For this review, take the finished solid that the model builds, in its own axes (mm). A direction names the side the tool comes from. Coordinates: 2 decimals unless noted, no trailing zeros. Write each loop counter-clockwise with the first axis right and the second up, starting at its lowest first coordinate (ties: lowest second). Pieces come first, ordered by that corner, then holes. Notation, with made-up numbers: (36, 50.25) -> (44, 50.25) arc R20 ccw to (44, 69.25) -> close; hole circle Ø8 at (58, 87.5). An arc over 180 degrees is marked (long way). Put each result on its own line as item: value. Start each with the question number.
Item 1: Consider section B-B on y = -3.5. Give the boundary of the cut face in (x, z), and give its area (3 significant figures).
Item 2: Consider section C-C on z = -97.5. Give the boundary of the cut face in (x, y), and give its area (3 significant figures).
Item 3: To check wall thickness, follow L1, parallel to Y at x = 125, z = -45; L2, parallel to Z at x = 26, y = -8.5; L3, parallel to Y at x = 14, z = -9. State the ranges of each line that lie inside material, in increasing order.
Item 4: Consider section A-A on x = 125.5. Give the boundary of the cut face in (y, z), and give its area (3 significant figures).
Item 5: Consider section D-D on x = 147. Give the boundary of the cut face in (y, z), and give its area (3 significant figures).
Item 6: Insertion check: P1, Ø6, axis at x = 101, y = -26, coming from the -Z side; P2, Ø6, axis at x = 33.5, z = -93.5, coming from the -Y side; P3, Ø5, axis at x = 147.5, y = -5, coming from the +Z side. Each pin has a flat end and moves straight along its axis. Give the tip position at first contact, or say it passes through.
Item 7: For faces 1 (the flat face through (43, -35, -10)), 2 (the flat face through (172.35, 4.93, -55.95)), list the 3-axis set-ups (+Z, -Z, +X, -X, +Y, -Y) from which the entire face can be reached by the end or side of a thin tool; tool diameter is ignored.
```python
from build123d import *

# Parameters (mm, degrees)
BOSS_EXTRUDE3_DEPTH = 10
BOSS_EXTRUDE4_DEPTH = 10


with BuildPart() as part:
    # Sketch3 → Boss-Extrude3 (new body)
    with BuildSketch(Plane.XY):
        Polygon((0, 0), (151.986841536, 0), (0, -130), align=None)
    extrude(amount=-BOSS_EXTRUDE3_DEPTH)

    # Sketch5 → Boss-Extrude4 (add)
    with BuildSketch(Plane(origin=(0, 0, 0), x_dir=(1, 0, 0), z_dir=(0, 1, 0))):
        with BuildLine():
            Line((0, 0), (151.986841536, 0))
            Line((151.986841536, 0), (193.295480236, 113.494552057))
            ThreePointArc((193.295480236, 113.494552057), (192.332468486, 122.287749574), (184.770111455, 126.876700471))
            Line((184.770111455, 126.876700471), (34.770111455, 140))
            ThreePointArc((34.770111455, 140), (12.126197015, 132.448649393), (2.162345286, 110.757835303))
            Line((2.162345286, 110.757835303), (0, 10))
            Line((0, 10), (0, 0))
        make_face()
    extrude(amount=BOSS_EXTRUDE4_DEPTH)


solid = part.part
```
Return value:
1. outline: (0, -10) -> (147.89, -10) -> (147.89, 0) -> (0, 0) -> close
1. area: 1,480 mm^2
2. outline: (1.88, 0) -> (187.47, 0) -> (187.47, 10) -> (1.88, 10) -> close
2. area: 1,860 mm^2
3. L1: 0 to 10
3. L2: -10 to 0
3. L3: -118.03 to 10
4. outline: (-22.66, -10) -> (0, -10) -> (0, -132.06) -> (10, -132.06) -> (10, 0) -> (-22.66, 0) -> close
4. area: 1,550 mm^2
5. outline: (-4.27, -10) -> (0, -10) -> (0, -130.18) -> (10, -130.18) -> (10, 0) -> (-4.27, 0) -> close
5. area: 1,340 mm^2
6. P1: z = -10
6. P2: y = 0
6. P3: z = 0
7. face 1: -Z, +X, -X, -Y
7. face 2: +Z, +X, +Y, -Y
